from build123d import *

# Parameters (mm, degrees)
F0_W      = 500
F0_H      = 42.25
F4_W      = 21
F4_H      = 28
F5_DEPTH  = 20
F7_DEPTH  = 15
F8_R      = 7.5
F9_DEPTH  = 3
F10_W     = 2
F10_H     = 2.5
F12_R     = 3
F13_DEPTH = 25


# Not quite as in the source:
# - a pattern or mirror of a feature is missing from the dataset's text; its kind, count and spacing are read off the source's solid


with BuildPart() as f1:
    # F0 (on Front) → F1 (revolve)
    with BuildSketch(Plane.XZ):
        with Locations((0, 21.125)):
            Rectangle(F0_W, F0_H)
        with BuildLine():
            ThreePointArc((250, 42.25), (0, 42.75), (-250, 42.25))
            Line((-250, 42.25), (250, 42.25))
        make_face()
    revolve(axis=Axis((0, 0, 0), (1, 0, 0)))

    # F2 (on Front) → F3 (revolve)
    with BuildSketch(Plane.XZ):
        Polygon((-253, 0), (-250, 0), (-250, 22.5), (-253, 19.5), align=None)
    f3 = revolve(axis=Axis((-251.5, 0, 0), (-1, 0, 0)))

    # F3_copies: F3 across plane
    add(f3.mirror(Plane(origin=(0, 0, 0), x_dir=(0, 0, 1), z_dir=(1, 0, 0))))

    # F4 (on face) → F5 (join)
    with BuildSketch(Plane(origin=(-253, 0, 0), x_dir=(0, -1, 0), z_dir=(-1, 0, 0))):
        Rectangle(F4_W, F4_H)
        with BuildLine():
            ThreePointArc((10.5, 14), (0, 17.5), (-10.5, 14))
            Line((-10.5, 14), (10.5, 14))
        make_face()
        with BuildLine():
            Line((10.5, -14), (-10.5, -14))
            ThreePointArc((-10.5, -14), (0, -17.5), (10.5, -14))
        make_face()
    f5 = extrude(amount=F5_DEPTH)

    # F5_copies: F5 across plane
    add(f5.mirror(Plane(origin=(0, 0, 0), x_dir=(0, 0, 1), z_dir=(1, 0, 0))))

    # F6 (on face) → F7 (join)
    with BuildSketch(Plane(origin=(-273, 0, 0), x_dir=(0, -1, 0), z_dir=(-1, 0, 0))):
        Polygon((0, 10), (-8.6602540378, 5), (-8.6602540378, -5), (0, -10), (8.6602540378, -5), (8.6602540378, 5), align=None)
    extrude(amount=F7_DEPTH)

    # F8 (on face) → F9 (cut)
    with BuildSketch(Plane(origin=(-288, 0, 0), x_dir=(0, -1, 0), z_dir=(-1, 0, 0))):
        Polygon((0, 10), (-8.6602540378, 5), (-8.6602540378, -5), (0, -10), (8.6602540378, -5), (8.6602540378, 5), align=None)
        Circle(F8_R, mode=Mode.SUBTRACT)
    extrude(amount=-F9_DEPTH, mode=Mode.SUBTRACT)

    # F10 (on Front) → F11 (revolve, cut)
    with BuildSketch(Plane.XZ):
        with Locations((-281, 8.75)):
            Rectangle(F10_W, F10_H)
    revolve(axis=Axis((-10, 0, 0), (-1, 0, 0)), mode=Mode.SUBTRACT)

    # F12 (on face) → F13 (join)
    with BuildSketch(Plane(origin=(-288, 0, 0), x_dir=(0, -1, 0), z_dir=(-1, 0, 0))):
        Circle(F12_R)
    extrude(amount=F13_DEPTH)


solid = f1.part
Design review of the part built by this model. Coordinates are the model's own, in mm. A direction names the side the tool comes from. Round coordinates to 2 decimals unless told otherwise and drop trailing zeros. One line per question, with ' | ' between items.
(1) Machinability: for faces 1 (the cylindrical face through (262.9, -0.2, 17.5)), 2 (the cylindrical face through (-262.9, -0.2, 17.5)), 3 (the flat face through (263, -10.5, 0)), 4 (the flat face through (-263, 10.5, 0)), which of the approach directions +Z, -Z, +X, -X, +Y, -Y give a long, thin tool a straight path to every point of the face, cutting with its end or side? Answer none if there is none.
Result sheet:
face 1: +Z, +X | face 2: +Z, -X | face 3: +Z, -Z, +X, -Y | face 4: +Z, -Z, -X, +Y
(2) Wall thickness on line 1 (X direction, y = 19.5, z = -2); line 2 (X direction, y = -5, z = 16.5); line 3 (Z direction, x = 19, y = -1): over which ranges is each line inside the solid? List them lowest first. Write a range as [from, to].
Result sheet:
line 1: [-252.9, 252.9] | line 2: [-273, 273] | line 3: [-42.74, 42.74]
(3) Insertion check: P1, Ø5.5, axis at x = -277.5, z = 1.5, coming from the -Y side; P2, Ø1, axis at y = -33, z = -19, coming from the +X side; P3, Ø3.5, axis at x = -276, z = 0, coming from the +Y side; P4, Ø4.5, axis at y = 3, z = -2, coming from the -X side. Each pin has a flat end and moves straight along its axis. Give the tip position at first contact, or say it passes through.
Result sheet:
P1: y = -8.66 | P2: x = 250 | P3: y = 8.66 | P4: x = -313
(4) Draft analysis for pull direction X (two halves, no side actions). For faces 5 (the flat face through (-273, 5, 8)), 6 (the flat face through (-282, 2, -7.4)), 7 (the cylindrical face through (-262.9, 0.2, -17.5)), state which applies: released by +X, released by -X, zero draft, split by the parting line, or undercut.
Result sheet:
face 5: released by -X | face 6: undercut | face 7: zero draft
